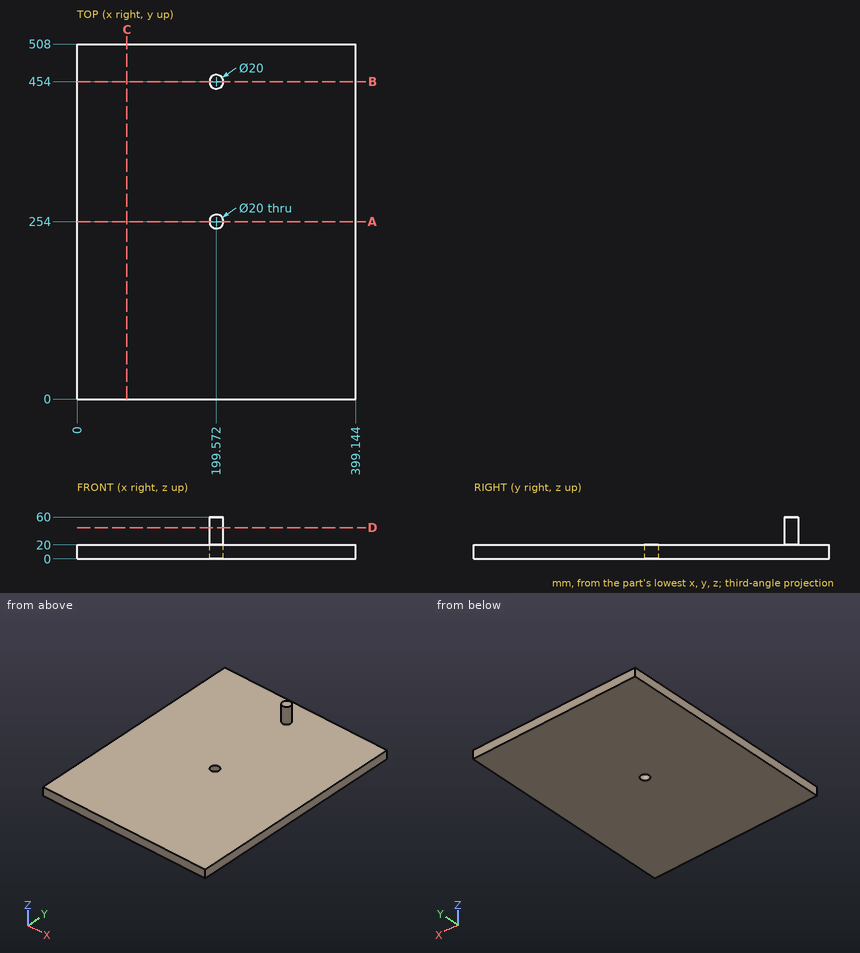
Answer from the drawing. Dimensions are ordinates in mm from the lowest x, y and z of the part. Coordinates: 2 decimals unless noted, no trailing zeros. Write each loop counter-clockwise with the first axis right and the second up, starting at its lowest first coordinate (ties: lowest second). Pieces come first, ordered by that corner, then holes. Notation, with made-up numbers: M 42.25,47.25 L 75.25,47.25 A17 ccw 75.25,76.25 Z; hole C 53.25,3 d5. An arc over 180 degrees is marked long. Use a Markdown table: item, result.
Q1. This flat-tipped pin is pushed along its axis until it touches: pin 1 Ø1 at (x, y) = (256.5, 231) entering from +Z. Where does it stop, or does it pass through?
Answer block:
| item | result |
|---|---|
| pin 1 | stops at z = 20 |
Q2. The part is cut by section B-B, the plane y = 454. Write down the section's boundary in (x, z), then the cut area to 3 significant figures.
Answer block:
| item | result |
|---|---|
| outline | M 0,0 L 399.14,0 L 399.14,20 L 209.57,20 L 209.57,60 L 189.57,60 L 189.57,20 L 0,20 Z |
| area | 8,780 mm2 |
Q3. The part is cut by section A-A, the plane y = 254. Write down the section's boundary in (x, z), then the cut area to 3 significant figures.
Answer block:
| item | result |
|---|---|
| outline | M 0,0 L 189.57,0 L 189.57,20 L 0,20 Z; M 209.57,0 L 399.14,0 L 399.14,20 L 209.57,20 Z |
| area | 7,580 mm2 |
Q4. The part is cut by section C-C, the plane x = 71.5. Write down the section's boundary in (y, z), then the cut area to 3 significant figures.
Answer block:
| item | result |
|---|---|
| outline | M 0,0 L 508,0 L 508,20 L 0,20 Z |
| area | 10,200 mm2 |
Q5. The part is cut by section D-D, the plane z = 45. Write down the section's boundary in (x, y), then the cut area to 3 significant figures.
Answer block:
| item | result |
|---|---|
| outline | C 199.57,454 d20 |
| area | 314 mm2 |
Q6. Straight lines are drawn through the part: L1, parallel to Z at x = 92.5, y = 57.5; L2, parallel to X at y = 452, z = 27.5; L3, parallel to X at y = 451.5, z = 55.5 (1 decimal). For each, find the intervals that lie inside material, in ascending order. Write a range as [from, to].
Answer block:
| item | result |
|---|---|
| L1 | z = [0, 20] |
| L2 | x = [189.77, 209.37] |
| L3 | x = [189.9, 209.3] |
